Geometry check sheet. Reference: the model listing, model coordinates, mm. A direction names the side the tool comes from. Round coordinates to 2 decimals unless told otherwise and drop trailing zeros. Write each question's results on one line, items separated by ' | '.
```python
from build123d import *

# Parameters (mm, degrees)
SKETCH1_R           = 3.05
BOSS_EXTRUDE1_DEPTH = 1.5
BOSS_EXTRUDE2_DEPTH = 49.25
CUT_EXTRUDE1_DEPTH  = 1
CUT_EXTRUDE3_DEPTH  = 64.82752638948185
SKETCH5_R           = 3.099999999999995
BOSS_EXTRUDE3_DEPTH = 0.5
CUT_EXTRUDE4_DEPTH  = 0.5
CHAMFER3_SIZE       = 1.5


with BuildPart() as part:
    # Sketch1 → Boss-Extrude1 (new body)
    with BuildSketch(Plane(origin=(0, 0, 0), x_dir=(1, 0, 0), z_dir=(0, 1, 0))):
        Polygon((-29.375, 24.624999999999996), (29.375, 24.624999999999996), (29.375000000000004, -24.625000000000004), (-29.374999999999993, -24.625000000000004), align=None)
        with Locations(Location((-3.47e-15, -3.47e-15, 0), (0, 0, 270))):
            Circle(SKETCH1_R, mode=Mode.SUBTRACT)
    extrude(amount=BOSS_EXTRUDE1_DEPTH)

    # Sketch2 → Boss-Extrude2 (add)
    with BuildSketch(Plane(origin=(0, 0, -24.624999999999996), x_dir=(-1, 0, 0), z_dir=(0, 0, -1))):
        Polygon((-29.375, 1.5), (29.375, 1.5), (29.375, 2.5), (28.199999999999996, 4), (27.025, 2.5), (25.849999999999998, 4), (24.675, 2.5), (23.499999999999996, 4), (22.325, 2.5), (21.149999999999995, 4), (19.974999999999998, 2.5), (18.799999999999997, 4), (17.625, 2.5), (16.45, 4), (15.275, 2.5), (14.099999999999998, 4), (12.924999999999999, 2.5), (11.749999999999998, 4), (10.575, 2.5), (9.399999999999999, 4), (8.225, 2.5), (7.049999999999999, 4), (5.874999999999999, 2.5), (4.699999999999999, 4), (3.525, 2.5), (2.3499999999999996, 4), (1.1749999999999996, 2.5), (0, 4), (-1.1749999999999996, 2.5), (-2.3499999999999996, 4), (-3.525, 2.5), (-4.699999999999999, 4), (-5.874999999999999, 2.5), (-7.049999999999999, 4), (-8.225, 2.5), (-9.399999999999999, 4), (-10.575, 2.5), (-11.749999999999998, 4), (-12.924999999999999, 2.5), (-14.099999999999998, 4), (-15.275, 2.5), (-16.45, 4), (-17.625, 2.5), (-18.799999999999997, 4), (-19.974999999999998, 2.5), (-21.149999999999995, 4), (-22.325, 2.5), (-23.499999999999996, 4), (-24.675, 2.5), (-25.849999999999998, 4), (-27.025, 2.5), (-28.199999999999996, 4), (-29.375, 2.5), align=None)
    extrude(amount=-BOSS_EXTRUDE2_DEPTH)

    # Sketch3 → Cut-Extrude1 (cut)
    with BuildSketch(Plane(origin=(0, 0, 0), x_dir=(-1, 0, 0), z_dir=(0, -1, 0))):
        with BuildLine():
            Line((-1.7499999999999998, -2.497999199359359), (-1.7499999999999993, -5))
            Line((-1.7499999999999993, -5), (1.7500000000000007, -5))
            Line((1.7500000000000007, -5), (1.7499999999999998, -2.4979991993593593))
            ThreePointArc((1.7499999999999998, -2.4979991993593593), (1.54e-15, 3.05), (-1.7499999999999998, -2.497999199359359))
        make_face()
    extrude(amount=-CUT_EXTRUDE1_DEPTH, mode=Mode.SUBTRACT)

    # Sketch4 → Cut-Extrude3 (cut, through all)
    with BuildSketch(Plane(origin=(29.375000000000004, 0, -4.14e-15), x_dir=(-1.4e-16, 0, -1), z_dir=(1, 0, -1.4e-16))):
        with BuildLine():
            Line((-23.875000000000007, 4), (-24.625000000000007, 4))
            Line((-24.625000000000007, 4), (-24.625000000000007, 3.2500000000000004))
            ThreePointArc((-24.625000000000007, 3.2500000000000004), (-24.40533008588992, 3.7803300858899114), (-23.875000000000007, 4))
        make_face()
    cut_extrude3 = extrude(amount=-CUT_EXTRUDE3_DEPTH, mode=Mode.SUBTRACT)

    # Mirror1: Cut-Extrude3 across plane
    add(cut_extrude3.mirror(Plane.XY), mode=Mode.SUBTRACT)

    # Sketch5 → Boss-Extrude3 (add)
    with BuildSketch(Plane.XZ.offset(-1.5)):
        Circle(SKETCH5_R)
    extrude(amount=BOSS_EXTRUDE3_DEPTH)

    # Sketch6 → Cut-Extrude4 (cut)
    with BuildSketch(Plane.XZ.offset(-1)):
        Polygon((1.7499999999999993, 5), (-1.7499999999999998, 5), (-1.7500000000000027, 2.497999199359363), (1.7499999999999993, 2.497999199359363), align=None)
    extrude(amount=-CUT_EXTRUDE4_DEPTH, mode=Mode.SUBTRACT)

    # Chamfer3
    chamfer3_edges = [part.edges().sort_by_distance(p)[0] for p in [
        (-6.7e-16, 0, 5),
    ]]
    chamfer(chamfer3_edges, length=CHAMFER3_SIZE - 0.0001)  # a hair under: the kernel refuses the full size


solid = part.part
```
(1) Material ranges on line 1 (X direction, y = 0.6, z = 0) (3 decimals); line 2 (X direction, y = 0.25, z = 5) (3 decimals); line 3 (Z direction, x = 0, y = 0.35) (3 decimals), recorded low to high.
Answers follow:
line 1: -29.375 to -3.05, 3.05 to 29.375 | line 2: -29.375 to -1.75, 1.75 to 29.375 | line 3: -24.625 to -3.05, 6.15 to 24.625
(2) Access from +Z, -Z, +X, -X, +Y, -Y to the whole of each face (thin tool, end or side, straight path). Record for faces 3 (the face through (0.11, 0.49, -3.05)), 4 (the face through (-15.9, 3.3, -0.3)).
Answers follow:
face 3: -Y | face 4: +Z, -Z, +Y
(3) Draft check along X on faces 1 (the face through (-22.92, 3.26, -0.34)), 2 (the face through (-1.8, 3.3, -0.3)). Enter one of: released by +X, released by -X, zero draft, split by the parting line, or undercut.
Answers follow:
face 1: undercut | face 2: undercut
(4) Depth check by flat-ended pin: pin 1 Ø3 at (x, z) = (-18.5, 18) entering from +Y. Enter the tip coordinate at first touch or a pass-through.
Answers follow:
pin 1: y = 4
